The listing builds one solid part. Answer for the finished solid, in the listing's coordinates (mm). Face numbers are marked on the shaded views. A direction names the side the tool comes from. Give positions to 0.01 mm unless a question says otherwise; leave off trailing zeros. Loops run counter-clockwise (first coordinate to the right, second up) from the corner with the lowest first, then second, coordinate; pieces in that order, holes last.
Item 1: The mould has two halves that part along X. Classify the marked faces 1, 2 and 3: pulls with the +X half, pulls with the -X half, needs draft (parallel to the pull), parting line crosses it, or undercut.
Item 2: Section A-A, the plane x = -22 is taken. Give the vertices of the cut face in (y, z), and give its area (3 significant figures).
Item 3: Section B-B, the plane y = 0 is taken. Give the vertices of the cut face in (x, z).
Item 4: Each of these flat-tipped pins is pushed along its axis until it touches: pin 1 Ø7 at (x, y) = (-27.5, 3) entering from +Z; pin 2 Ø4 at (x, y) = (22, 0) entering from -Z; pin 3 Ø1.5 at (y, z) = (-2, -3) entering from -X; pin 4 Ø5 at (y, z) = (-3.5, -4) entering from -X. Where does it stop, or does it pass through?
Item 5: A tool of negligible diameter and unlimited length cuts with its end or side. For the marked faces 4, 5, 6 and 7, from which of +Z, -Z, +X, -X, +Y, -Y can it reach the whole face along a straight path? Write none if from no direction.
Item 6: Section D-D, the plane y = 5.5 is taken. Give the vertices of the cut face in (x, z), and give its area (3 significant figures).
Item 7: Section C-C, the plane z = -16 is taken. Give the vertices of the cut face in (x, y), and give its area (3 significant figures).
Item 8: Consider line 1 along Y through (x, z) = (-22, -18.65); line 2 along X through (y, z) = (4.75, -14.25); line 3 along Z through (x, y) = (-5, -5.75). Determine where each line is inside the solid, lowest interval first.
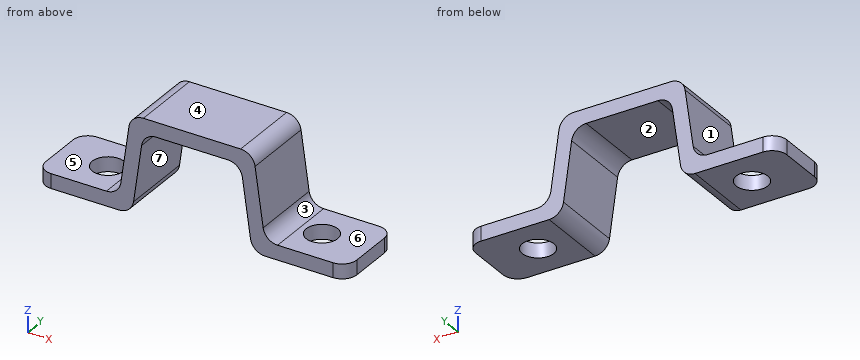
from build123d import *

# Parameters (mm, degrees)
EXTRUDE_1_DEPTH     = 7.5
SKETCH_2_R          = 3.25
CUT_EXTRUDE_1_DEPTH = 38.003378224
FILLET_1_R          = 3
FILLET_2_R          = 3


with BuildPart() as part:
    # 草图1 → 凸台-拉伸1 (new, symmetric)
    with BuildSketch(Plane(origin=(0, 0, 0), x_dir=(1, 0, 0), z_dir=(0, 1, 0))):
        Polygon((-12.607332667, 0), (12.607332667, 0), (15, 17), (32, 17), (32, 20), (12.392667333, 20), (10, 3), (-10, 3), (-12.392667333, 20), (-32, 20), (-32, 17), (-15, 17), align=None)
    extrude(amount=EXTRUDE_1_DEPTH, both=True)

    # 草图2 → 切除-拉伸1 (cut, through all)
    with BuildSketch(Plane.XY.offset(-17)):
        with Locations((-22, 0)):
            Circle(SKETCH_2_R)
        with Locations(Location((22, 0, 0), (0, 0, 180))):
            Circle(SKETCH_2_R)
    extrude(amount=-CUT_EXTRUDE_1_DEPTH, mode=Mode.SUBTRACT)

    # 圆角1
    fillet_1_edges = [part.edges().sort_by_distance(p)[0] for p in [
        (15, 0, -17),
        (12.607332667, 0, 0),
        (-12.607332667, 0, 0),
        (-15, 0, -17),
        (-12.392667333, 0, -20),
        (-10, 0, -3),
        (10, 0, -3),
        (12.392667333, 0, -20),
    ]]
    fillet(fillet_1_edges, radius=FILLET_1_R)

    # 圆角2
    fillet_2_edges = [part.edges().sort_by_distance(p)[0] for p in [
        (-32, -7.5, -18.5),
        (32, -7.5, -18.5),
        (-32, 7.5, -18.5),
        (32, 7.5, -18.5),
    ]]
    fillet(fillet_2_edges, radius=FILLET_2_R)


solid = part.part
Worked answers:
1. face 1: pulls with the -X half
1. face 2: undercut
1. face 3: pulls with the +X half
2. outline: (-7.5, -20) - (-3.25, -20) - (-3.25, -17) - (-7.5, -17) - close; (3.25, -20) - (7.5, -20) - (7.5, -17) - (3.25, -17) - close
2. area: 25.5 mm2
3. outline: (-32, -20) - (-25.25, -20) - (-25.25, -17) - (-32, -17) - close; (-18.75, -20) - (-15, -20) arc R3 ccw to (-12.03, -17.42) - (-10.36, -5.58) arc R3 cw to (-7.39, -3) - (7.39, -3) arc R3 cw to (10.36, -5.58) - (12.03, -17.42) arc R3 ccw to (15, -20) - (18.75, -20) - (18.75, -17) - (17.61, -17) arc R3 cw to (14.64, -14.42) - (12.97, -2.58) arc R3 ccw to (10, 0) - (-10, 0) arc R3 ccw to (-12.97, -2.58) - (-14.64, -14.42) arc R3 cw to (-17.61, -17) - (-18.75, -17) - close; (25.25, -20) - (32, -20) - (32, -17) - (25.25, -17) - close
4. pin 1: stops at z = -17
4. pin 2: passes through
4. pin 3: stops at x = -13.14
4. pin 4: stops at x = -13.52
5. face 4: +Z, +X, -X, +Y, -Y
5. face 5: +Z, -X, +Y, -Y
5. face 6: +Z, +X, +Y, -Y
5. face 7: -Z, +Y, -Y
6. outline: (-31.83, -20) - (-15, -20) arc R3 ccw to (-12.03, -17.42) - (-10.36, -5.58) arc R3 cw to (-7.39, -3) - (7.39, -3) arc R3 cw to (10.36, -5.58) - (12.03, -17.42) arc R3 ccw to (15, -20) - (31.83, -20) - (31.83, -17) - (17.61, -17) arc R3 cw to (14.64, -14.42) - (12.97, -2.58) arc R3 ccw to (10, 0) - (-10, 0) arc R3 ccw to (-12.97, -2.58) - (-14.64, -14.42) arc R3 cw to (-17.61, -17) - (-31.83, -17) - close
6. area: 280 mm2
7. outline: (-15.37, -7.5) - (-11.83, -7.5) - (-11.83, 7.5) - (-15.37, 7.5) - close; (11.83, -7.5) - (15.37, -7.5) - (15.37, 7.5) - (11.83, 7.5) - close
7. area: 106 mm2
8. line 1: y = -7.5 to -3.25, 3.25 to 7.5
8. line 2: x = -14.61 to -11.58, 11.58 to 14.61
8. line 3: z = -3 to 0
